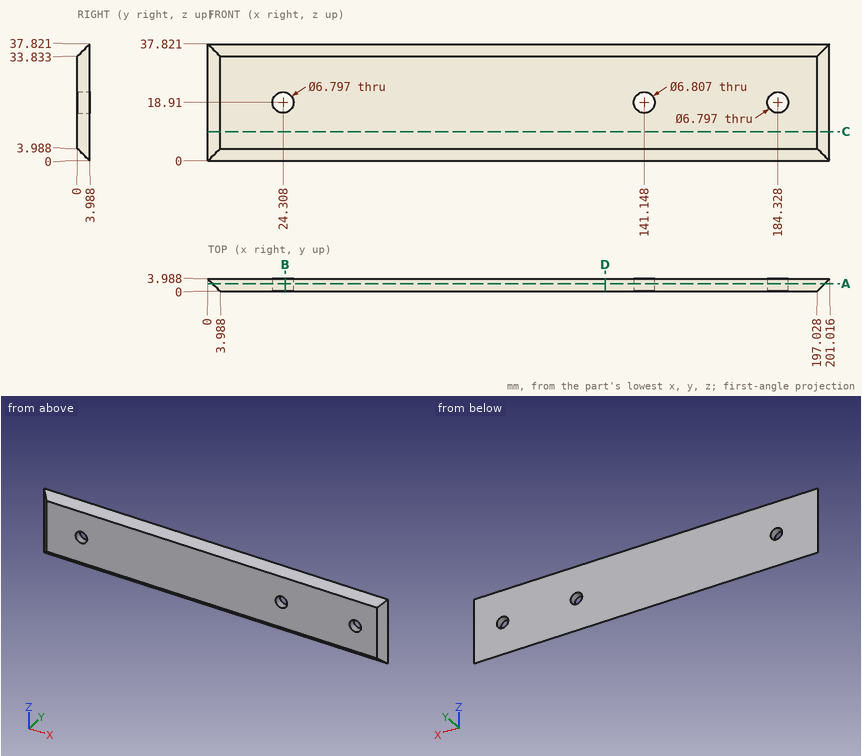
Geometry: see drawing. Coordinates: mm, zero at the bounding-box minimum. Round coordinates to 2 decimals unless told otherwise and drop trailing zeros. Write each loop counter-clockwise with the first axis right and the second up, starting at its lowest first coordinate (ties: lowest second). Pieces come first, ordered by that corner, then holes.
1) Cut plane C-C (z = 9.5). Return the cut outline in (x, y) (1 decimal).
2) Ray query, L1, parallel to X at y = 3, z = 18 (1 decimal); L2, parallel to X at y = 2.6, z = 18 (1 decimal); L3, parallel to Z at x = 181.5, y = 2.9 (1 decimal). Return the intervals inside material, ascending.
3) Contact query for flat-ended pins moving along their axis: P1, Ø2, axis at x = 58, y = 1.5, coming from the -Z side; P2, Ø5.5, axis at x = 184.33, z = 18.91, coming from the -Y side; P3, Ø2, axis at y = 0.5, z = 28.5, coming from the -X side. Output: stop coordinate, or through.
4) Cut plane A-A (y = 2.45). Return the cut outline in (x, z) (1 decimal), then the cut area to 3 significant figures.
5) Cut plane D-D (x = 128.5). Return the cut outline in (y, z), then the cut area to 3 significant figures.
6) Cut plane B-B (x = 25). Return the cut outline in (y, z).
Geometry says:
1. outline: (0, 4) - (4, 0) - (197, 0) - (201, 4) - close
2. L1: x = 1 to 21, 27.6 to 137.9, 144.4 to 181.1, 187.6 to 200
2. L2: x = 1.4 to 21, 27.6 to 137.9, 144.4 to 181.1, 187.6 to 199.6
2. L3: z = 1.1 to 17, 20.8 to 36.7
3. P1: stops at z = 1.49
3. P2: passes through
3. P3: stops at x = 2.49
4. outline: (1.5, 1.5) - (199.5, 1.5) - (199.5, 36.3) - (1.5, 36.3) - close; hole circle Ø6.8 at (24.3, 18.9); hole circle Ø6.8 at (141.1, 18.9); hole circle Ø6.8 at (184.3, 18.9)
4. area: 6,770 mm2
5. outline: (0, 3.99) - (3.99, 0) - (3.99, 37.82) - (0, 33.83) - close
5. area: 135 mm2
6. outline: (0, 3.99) - (3.99, 0) - (3.99, 15.58) - (0, 15.58) - close; (0, 22.24) - (3.99, 22.24) - (3.99, 37.82) - (0, 33.83) - close
